Read the model definition and answer for the solid it produces. Units are mm, in the model's axes. Coordinates: 2 decimals unless noted, no trailing zeros. Order: outer loops, then holes, each group sorted by start corner. A loop starts at its lowest first (then second) coordinate and runs counter-clockwise, first axis right, second up. Notation, with made-up numbers: (-23.5, 52) -> (30.5, 52) arc R7 cw to (30.5, 57) -> close; hole circle Ø1 at (19, 36.25). An arc over 180 degrees is marked (long way). Answer in a Markdown table with one row per item.
from build123d import *

# Parameters (mm, degrees)
F0_R     = 1.5
F1_DEPTH = 3
F2_R     = 12
F2_R_2   = 1.5
F3_DEPTH = 25
F4_R     = 2.1
F5_DEPTH = 25


with BuildPart() as f1:
    # F0 (on Front) → F1 (new body)
    with BuildSketch(Plane.XZ):
        with BuildLine():
            Line((-102, -16.5), (-102, -23))
            Line((-102, -23), (0, -23))
            Line((0, -23), (102, -23))
            Line((102, -23), (102, -16.5))
            Line((102, -16.5), (100, -16.5))
            Line((100, -16.5), (100, 42.5))
            Line((100, 42.5), (104.5, 42.5))
            ThreePointArc((104.5, 42.5), (102.596194, 47.096194), (98, 49))
            ThreePointArc((98, 49), (94.28238, 50.068786), (91.7, 52.948771))
            ThreePointArc((91.7, 52.948771), (90.347923, 54.513813), (88.394881, 55.194327))
            ThreePointArc((88.394881, 55.194327), (44.227467, 57.601774), (0, 58.3))
            ThreePointArc((0, 58.3), (-44.227467, 57.601774), (-88.394881, 55.194327))
            ThreePointArc((-88.394881, 55.194327), (-90.347923, 54.513813), (-91.7, 52.948771))
            ThreePointArc((-91.7, 52.948771), (-94.28238, 50.068786), (-98, 49))
            ThreePointArc((-98, 49), (-102.596194, 47.096194), (-104.5, 42.5))
            Line((-104.5, 42.5), (-102, 42.5))
            Line((-102, 42.5), (-100, 42.5))
            Line((-100, 42.5), (-100, -16.5))
            Line((-100, -16.5), (-102, -16.5))
        make_face()
        with Locations((-94.5, -17.5)):
            Circle(F0_R, mode=Mode.SUBTRACT)
        with Locations((94.5, -17.5)):
            Circle(F0_R, mode=Mode.SUBTRACT)
        with Locations((-86.5, 49.5)):
            Circle(F0_R, mode=Mode.SUBTRACT)
        with Locations((86.5, 49.5)):
            Circle(F0_R, mode=Mode.SUBTRACT)
    extrude(amount=F1_DEPTH)

    # F2 (on face) → F3 (cut)
    with BuildSketch(Plane.XZ.offset(3)):
        with Locations((78, 27)):
            Circle(F2_R)
        with Locations((87.5, 15)):
            Circle(F2_R_2)
        with Locations((68.5, 39)):
            Circle(F2_R_2)
    extrude(amount=-F3_DEPTH, mode=Mode.SUBTRACT)

    # F4 (on face) → F5 (cut)
    with BuildSketch(Plane.XZ.offset(3)):
        with BuildLine():
            Line((15.25, 39.65), (-47.75, 39.65))
            ThreePointArc((-47.75, 39.65), (-57.225231, 35.725231), (-61.15, 26.25))
            Line((-61.15, 26.25), (-61.15, 15.25))
            ThreePointArc((-61.15, 15.25), (-57.225231, 5.774769), (-47.75, 1.85))
            Line((-47.75, 1.85), (15.25, 1.85))
            ThreePointArc((15.25, 1.85), (24.725231, 5.774769), (28.65, 15.25))
            Line((28.65, 15.25), (28.65, 26.25))
            ThreePointArc((28.65, 26.25), (24.725231, 35.725231), (15.25, 39.65))
        make_face()
        with Locations((-76, 38.5)):
            Circle(F4_R)
        with Locations((-76, 3)):
            Circle(F4_R)
        with Locations((43.5, 3)):
            Circle(F4_R)
        with Locations((43.5, 38.5)):
            Circle(F4_R)
    extrude(amount=-F5_DEPTH, mode=Mode.SUBTRACT)


solid = f1.part
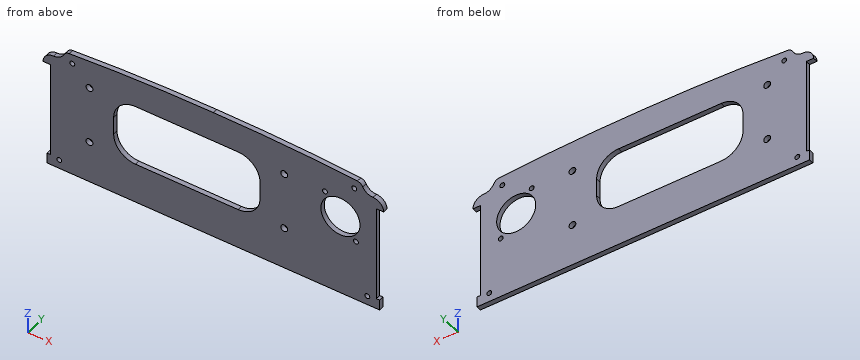
Q1. The part is cut by section B-B (z = 33). Write down the section's boundary in (x, y).
Outcome:
| item | result |
|---|---|
| outline | (-100, -3) -> (-59.33, -3) -> (-59.33, 0) -> (-100, 0) -> close; (26.83, -3) -> (67.61, -3) -> (67.61, 0) -> (26.83, 0) -> close; (88.39, -3) -> (100, -3) -> (100, 0) -> (88.39, 0) -> close |
Q2. The part is cut by section C-C (x = -53). Write down the section's boundary in (y, z).
Outcome:
| item | result |
|---|---|
| outline | (-3, -23) -> (0, -23) -> (0, 2.92) -> (-3, 2.92) -> close; (-3, 38.58) -> (0, 38.58) -> (0, 57.26) -> (-3, 57.26) -> close |
Q3. Consider line 1 (X direction, y = -1.1, z = 35); line 2 (Z direction, x = 43.5, y = -1.3); line 3 (X direction, y = -2.2, z = -10.5). Determine where each line is inside the solid, lowest interval first.
Outcome:
| item | result |
|---|---|
| line 1 | -100 to -57.9, 25.4 to 69.06, 86.94 to 100 |
| line 2 | -23 to 0.9, 5.1 to 36.4, 40.6 to 57.63 |
| line 3 | -100 to 100 |
Q4. The part is cut by section D-D (y = -1.95). Give the number of separate pieces and of enclosed holes in the cut face, then the cut area to 3 significant figures.
Outcome:
| item | result |
|---|---|
| separate pieces | 1 |
| enclosed holes | 12 |
| area | 12,200 mm² |
Q5. Given pin 1 (1 mm diameter, centred on y = -2.5, z = 6.5, fed in from -X); pin 2 (0.9 mm diameter, centred on y = -2, z = 22.5, fed in from +X); pin 3 (4 mm diameter, centred on x = -76, z = 38.5, fed in from +Y); pin 4 (0.6 mm diameter, centred on x = 100.5, y = -1, fed in from +Z), each flat-ended and moving along its own axis, determine where each tip first touches the part or whether it passes through.
Outcome:
| item | result |
|---|---|
| pin 1 | x = -100 |
| pin 2 | x = 100 |
| pin 3 | through |
| pin 4 | z = 48.62 |
Q6. The part is cut by section A-A (x = -76). Write down the section's boundary in (y, z).
Outcome:
| item | result |
|---|---|
| outline | (-3, -23) -> (0, -23) -> (0, 0.9) -> (-3, 0.9) -> close; (-3, 5.1) -> (0, 5.1) -> (0, 36.4) -> (-3, 36.4) -> close; (-3, 40.6) -> (0, 40.6) -> (0, 56.04) -> (-3, 56.04) -> close |
